Could you check a few things on this model? Use its own coordinates, in mm. Give positions to 0.01 mm unless a question says otherwise; leave off trailing zeros. Write each loop counter-clockwise with the first axis right and the second up, starting at its lowest first coordinate (ties: lowest second). Pieces come first, ordered by that corner, then holes. Notation, with made-up numbers: M 10.25,-31.5 L 48.25,-31.5 A22 cw 48.25,-14.5 Z; hole C 18,38.5 d2. An arc over 180 degrees is marked long. Write each question's results on one line, items separated by ' | '. Start each with the question number.
from build123d import *

# Parameters (mm, degrees)
SKETCH1_W           = 254
SKETCH1_H           = 72.69988
SKETCH1_R           = 1.5
SKETCH1_W_2         = 234.95
SKETCH1_H_2         = 53.64988
BOSS_EXTRUDE1_DEPTH = 3.175


with BuildPart() as part:
    # Sketch1 → Boss-Extrude1 (new body)
    with BuildSketch(Plane(origin=(0, 0, 0), x_dir=(1, 0, 0), z_dir=(0, 1, 0))):
        with Locations((127, 36.34994)):
            Rectangle(SKETCH1_W, SKETCH1_H)
        with Locations(Location((177.8, 67.93738, 0), (0, 0, 270))):
            Circle(SKETCH1_R, mode=Mode.SUBTRACT)
        with Locations(Location((177.8, 4.7625, 0), (0, 0, 90))):
            Circle(SKETCH1_R, mode=Mode.SUBTRACT)
        with Locations(Location((228.6, 67.93738, 0), (0, 0, 270))):
            Circle(SKETCH1_R, mode=Mode.SUBTRACT)
        with Locations(Location((228.6, 4.7625, 0), (0, 0, 90))):
            Circle(SKETCH1_R, mode=Mode.SUBTRACT)
        with Locations(Location((127, 67.93738, 0), (0, 0, 270))):
            Circle(SKETCH1_R, mode=Mode.SUBTRACT)
        with Locations(Location((127, 4.7625, 0), (0, 0, 90))):
            Circle(SKETCH1_R, mode=Mode.SUBTRACT)
        with Locations(Location((25.4, 4.7625, 0), (0, 0, 270))):
            Circle(SKETCH1_R, mode=Mode.SUBTRACT)
        with Locations(Location((76.2, 4.7625, 0), (0, 0, 270))):
            Circle(SKETCH1_R, mode=Mode.SUBTRACT)
        with Locations(Location((25.4, 67.93738, 0), (0, 0, 90))):
            Circle(SKETCH1_R, mode=Mode.SUBTRACT)
        with Locations(Location((76.2, 67.93738, 0), (0, 0, 90))):
            Circle(SKETCH1_R, mode=Mode.SUBTRACT)
        with Locations((127, 36.34994)):
            Rectangle(SKETCH1_W_2, SKETCH1_H_2, mode=Mode.SUBTRACT)
    extrude(amount=-BOSS_EXTRUDE1_DEPTH)


solid = part.part
Q1. If we section it at B-B (y = -1.9): Count the separate pieces of the cut face and the enclosed holes in it, plus the area to 3 significant figures.
Q2. Please list where these lines run through material, in increasing order: line 1 (Z direction, x = 127, y = -1.05) (1 decimal); line 2 (X direction, y = -1.1, z = -56) (3 decimals); line 3 (Z direction, x = 216, y = -0.5) (3 decimals). Write a range as [from, to].
Q3. If we section it at C-C (x = 135): Please give me the cut outline in (y, z) (3 decimals).
Q4. If we section it at A-A (z = -17): Please give me the cut outline in (x, y) (3 decimals), plus the area to 3 significant figures.
Determined:
1) separate pieces: 1 | enclosed holes: 11 | area: 5,790 mm²
2) line 1: z = [-72.7, -69.4], [-66.4, -63.2], [-9.5, -6.3], [-3.3, 0] | line 2: x = [0, 9.525], [244.475, 254] | line 3: z = [-72.7, -63.175], [-9.525, 0]
3) outline: M -3.175,-72.7 L 0,-72.7 L 0,-63.175 L -3.175,-63.175 Z; M -3.175,-9.525 L 0,-9.525 L 0,0 L -3.175,0 Z
4) outline: M 0,-3.175 L 9.525,-3.175 L 9.525,0 L 0,0 Z; M 244.475,-3.175 L 254,-3.175 L 254,0 L 244.475,0 Z | area: 60.5 mm²
